For this review, take the finished solid that the model builds, in its own axes (mm). A direction names the side the tool comes from. Give positions to 0.01 mm unless a question says otherwise; leave off trailing zeros. Order: outer loops, then holes, each group sorted by start corner. A loop starts at its lowest first (then second) coordinate and runs counter-clockwise, first axis right, second up. Notation, with made-up numbers: (-6, 4.5) - (51, 4.5) arc R35 ccw to (51, 43.5) - close; hole circle Ø11 at (55, 70). An arc over 180 degrees is marked (long way). Use a Markdown table: item, result. Add a question column.
1) We need section C-C on z = 2.5. Give the number of separate pieces and of enclosed holes in the cut face, then the cut area to 3 significant figures.
2) Wall thickness on L1, parallel to X at y = 116, z = 8.25; L2, parallel to Y at x = -66, z = 7.5; L3, parallel to Y at x = -77.5, z = 3.75: over which ranges is each line inside the solid? List them lowest first.
3) We need section D-D on y = 240. Write out the cut boundary in (x, z), then the cut area to 3 significant figures.
4) Clearance check with flat-ended pins moving along their axes: P1, Ø1, axis at x = -72, y = 142, coming from the -Z side; P2, Ø3, axis at x = -66, z = 4.5, coming from the +Y side; P3, Ø3, axis at y = 59, z = 7.5, coming from the +X side. State where each tip first meets the part, or that it passes through.
5) We need section A-A on x = -92. Write out the cut boundary in (y, z), then the cut area to 3 significant figures.
6) We need section B-B on y = 135.5. Write out the cut boundary in (x, z).
7) Machinability: for faces 4 (the face through (-68, 89.953, 5)), 5 (the face through (-92, 34.953, 5)), 6 (the face through (-74.14, 233, 5)), 7 (the face through (-85, 104.953, 5)), 8 (the face through (-62.544, 148, 5)), which of the approach directions +Z, -Z, +X, -X, +Y, -Y give a long, thin tool a straight path to every point of the face, cutting with its end or side? Answer none if there is none.
8) Mouldability with a two-part tool opening along Y and no side actions: class faces 1 (the face through (-92, 259.953, 5)), 2 (the face through (-64.694, 147, 5)), 3 (the face through (-101, 149, 0)) as released by +Y, released by -Y, zero draft, split by the parting line, or undercut.
```python
from build123d import *

# Parameters (mm, degrees)
SKETCH4_R           = 1.6
SKETCH4_W           = 30
SKETCH4_H           = 85
BOSS_EXTRUDE6_DEPTH = 10


with BuildPart() as part:
    # Sketch4 → Boss-Extrude6 (new body)
    with BuildSketch(Plane.XY):
        Polygon((-109.544479684, 259.95267573), (-74.140420057, 259.95267573), (-74.140420057, 204.95267573), (-62.544479684, 204.95267573), (-62.544479684, 89.95267573), (-74.140420057, 89.95267573), (-74.140420057, 34.95267573), (-109.544479684, 34.95267573), align=None)
        with Locations((-77.519250358, 254.723971913)):
            Circle(SKETCH4_R, mode=Mode.SUBTRACT)
        with Locations((-106.178709835, 40.181379546)):
            Circle(SKETCH4_R, mode=Mode.SUBTRACT)
        with Locations((-77.519250358, 40.181379546)):
            Circle(SKETCH4_R, mode=Mode.SUBTRACT)
        with Locations((-66.044479684, 94.019745429)):
            Circle(SKETCH4_R, mode=Mode.SUBTRACT)
        with Locations((-107.209755901, 147.45267573)):
            Circle(SKETCH4_R, mode=Mode.SUBTRACT)
        with Locations((-66.044479684, 200.885606031)):
            Circle(SKETCH4_R, mode=Mode.SUBTRACT)
        with Locations((-106.178709835, 254.723971913)):
            Circle(SKETCH4_R, mode=Mode.SUBTRACT)
        with Locations((-84.544479684, 147.45267573)):
            Rectangle(SKETCH4_W, SKETCH4_H, mode=Mode.SUBTRACT)
        with BuildLine():
            Line((-67.394479684, 189.95267573), (-67.394479684, 147.45267573))
            Line((-67.394479684, 147.45267573), (-67.394479684, 104.95267573))
            ThreePointArc((-67.394479684, 104.95267573), (-66.044479684, 103.60267573), (-64.694479684, 104.95267573))
            Line((-64.694479684, 104.95267573), (-64.694479684, 147.45267573))
            Line((-64.694479684, 147.45267573), (-64.694479684, 189.95267573))
            ThreePointArc((-64.694479684, 189.95267573), (-66.044479684, 191.30267573), (-67.394479684, 189.95267573))
        make_face(mode=Mode.SUBTRACT)
        with BuildLine():
            Line((-104.394479684, 189.95267573), (-104.394479684, 147.45267573))
            Line((-104.394479684, 147.45267573), (-104.394479684, 104.95267573))
            ThreePointArc((-104.394479684, 104.95267573), (-103.044479684, 103.60267573), (-101.694479684, 104.95267573))
            Line((-101.694479684, 104.95267573), (-101.694479684, 147.45267573))
            Line((-101.694479684, 147.45267573), (-101.694479684, 189.95267573))
            ThreePointArc((-101.694479684, 189.95267573), (-103.044479684, 191.30267573), (-104.394479684, 189.95267573))
        make_face(mode=Mode.SUBTRACT)
    extrude(amount=BOSS_EXTRUDE6_DEPTH)


solid = part.part
```
Checked values:
| question | item | result |
|---|---|---|
| 1 | separate pieces | 1 |
| 1 | enclosed holes | 10 |
| 1 | area | 6,220 mm² |
| 2 | L1 | -109.54 to -104.39, -101.69 to -99.54, -69.54 to -67.39, -64.69 to -62.54 |
| 2 | L2 | 89.95 to 92.42, 95.62 to 103.6, 191.3 to 199.29, 202.48 to 204.95 |
| 2 | L3 | 34.95 to 38.58, 41.78 to 104.95, 189.95 to 253.12, 256.32 to 259.95 |
| 3 | outline | (-109.54, 0) - (-74.14, 0) - (-74.14, 10) - (-109.54, 10) - close |
| 3 | area | 354 mm² |
| 4 | P1 | through |
| 4 | P2 | y = 204.95 |
| 4 | P3 | x = -74.14 |
| 5 | outline | (34.95, 0) - (104.95, 0) - (104.95, 10) - (34.95, 10) - close; (189.95, 0) - (259.95, 0) - (259.95, 10) - (189.95, 10) - close |
| 5 | area | 1,400 mm² |
| 6 | outline | (-109.54, 0) - (-104.39, 0) - (-104.39, 10) - (-109.54, 10) - close; (-101.69, 0) - (-99.54, 0) - (-99.54, 10) - (-101.69, 10) - close; (-69.54, 0) - (-67.39, 0) - (-67.39, 10) - (-69.54, 10) - close; (-64.69, 0) - (-62.54, 0) - (-62.54, 10) - (-64.69, 10) - close |
| 7 | face 4 | +Z, -Z, +X, -Y |
| 7 | face 5 | +Z, -Z, +X, -X, -Y |
| 7 | face 6 | +Z, -Z, +X, +Y |
| 7 | face 7 | +Z, -Z |
| 7 | face 8 | +Z, -Z, +X, +Y, -Y |
| 8 | face 1 | released by +Y |
| 8 | face 2 | undercut |
| 8 | face 3 | zero draft |
